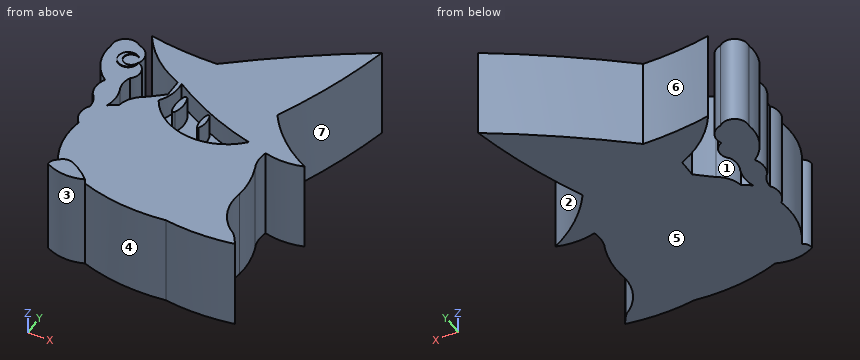
from build123d import *

# Parameters (mm, degrees)
F1_DEPTH = 25.4
F3_DEPTH = 0.254
F5_DEPTH = 6.35
F7_DEPTH = 1.27


with BuildPart() as f1:
    # F0 (on Top) → F1 (new body)
    with BuildSketch(Plane.XY):
        with BuildLine():
            ThreePointArc((25.499046, 10.18772), (37.34433, 7.273723), (49.542308, 7.166576))
            ThreePointArc((49.542308, 7.166576), (59.109263, 6.361494), (68.676218, 7.166576))
            ThreePointArc((68.676218, 7.166576), (67.66707, 8.882251), (66.488296, 10.486125))
            ThreePointArc((66.488296, 10.486125), (61.480718, 16.596846), (60.651142, 24.453597))
            ThreePointArc((60.651142, 24.453597), (60.581585, 29.680598), (59.400324, 34.772847))
            ThreePointArc((59.400324, 34.772847), (58.595793, 37.960262), (58.879148, 41.23541))
            ThreePointArc((58.879148, 41.23541), (64.299362, 40.444263), (69.719575, 41.23541))
            ThreePointArc((69.719575, 41.23541), (61.198485, 47.34438), (54.501284, 55.41135))
            ThreePointArc((54.501284, 55.41135), (61.017596, 71.57709), (65.758646, 88.349566))
            ThreePointArc((65.758646, 88.349566), (48.603509, 77.579957), (32.279015, 65.588541))
            ThreePointArc((32.279015, 65.588541), (22.727137, 66.05081), (13.27099, 67.476757))
            ThreePointArc((13.27099, 67.476757), (19.281494, 60.099473), (27.243776, 54.888662))
            Line((27.243776, 54.888662), (27.243776, 49.727544))
            ThreePointArc((27.243776, 49.727544), (24.946398, 47.862182), (22.58618, 46.076994))
            ThreePointArc((22.58618, 46.076994), (19.956312, 43.712231), (18.683871, 40.412351))
            ThreePointArc((18.683871, 40.412351), (17.413772, 39.740532), (16.166251, 39.027661))
            ThreePointArc((16.166251, 39.027661), (16.709722, 42.300567), (16.166251, 45.573473))
            ThreePointArc((16.166251, 45.573473), (15.61028, 48.154032), (16.166251, 50.734591))
            ThreePointArc((16.166251, 50.734591), (17.468425, 54.06764), (15.285085, 56.902759))
            ThreePointArc((15.285085, 56.902759), (15.245628, 60.550066), (12.389823, 62.819161))
            ThreePointArc((12.389823, 62.819161), (8.109951, 63.436313), (6.221656, 59.546258))
            ThreePointArc((6.221656, 59.546258), (6.981172, 52.747617), (11.148616, 47.322601))
            ThreePointArc((11.148616, 47.322601), (10.300829, 44.357989), (10.931111, 41.339643))
            ThreePointArc((10.931111, 41.339643), (12.26077, 39.219384), (12.659186, 36.748603))
            ThreePointArc((12.659186, 36.748603), (11.67473, 33.258245), (13.162711, 29.95103))
            ThreePointArc((13.162711, 29.95103), (13.136507, 21.545797), (16.183855, 13.712387))
            ThreePointArc((16.183855, 13.712387), (15.066637, 12.687257), (14.799166, 11.194767))
            ThreePointArc((14.799166, 11.194767), (20.034555, 9.474147), (25.499046, 10.18772))
        make_face()
    extrude(amount=F1_DEPTH)

    # F2 (on face) → F3 (join)
    with BuildSketch(Plane.XY.offset(25.4)):
        with BuildLine():
            ThreePointArc((15.285085, 56.902759), (11.304381, 56.052081), (14.373336, 58.726248))
            ThreePointArc((14.373336, 58.726248), (10.050782, 55.425279), (15.285085, 56.902759))
        make_face()
    extrude(amount=F3_DEPTH)

    # F4 (on face) → F5 (cut)
    with BuildSketch(Plane.XY.offset(25.4)):
        with BuildLine():
            ThreePointArc((28.30782, 54.837245), (28.14811, 50.533264), (26.335881, 46.626144))
            ThreePointArc((26.335881, 46.626144), (38.875379, 37.904283), (53.269263, 43.01564))
            ThreePointArc((53.269263, 43.01564), (40.303335, 47.901924), (28.30782, 54.837245))
        make_face()
        with BuildLine():
            ThreePointArc((39.436687, 42.002268), (39.013767, 44.590738), (39.47692, 47.172312))
            ThreePointArc((39.47692, 47.172312), (39.828965, 47.383895), (40.181011, 47.172312))
            ThreePointArc((40.181011, 47.172312), (40.563597, 44.57128), (39.919492, 42.022385))
            ThreePointArc((39.919492, 42.022385), (39.683239, 41.888733), (39.436687, 42.002268))
        make_face(mode=Mode.SUBTRACT)
        with BuildLine():
            ThreePointArc((31.047942, 44.697933), (30.682425, 47.680975), (31.24911, 50.632417))
            ThreePointArc((31.24911, 50.632417), (31.716176, 50.937117), (32.15437, 50.592184))
            ThreePointArc((32.15437, 50.592184), (32.630986, 47.625359), (31.953201, 44.697933))
            ThreePointArc((31.953201, 44.697933), (31.500571, 44.415393), (31.047942, 44.697933))
        make_face(mode=Mode.SUBTRACT)
    extrude(amount=-F5_DEPTH, mode=Mode.SUBTRACT)

    # F6 (on face) → F7 (join)
    with BuildSketch(Plane.XY.offset(25.4)):
        with BuildLine():
            ThreePointArc((19.70306, 14.540644), (17.799455, 14.738373), (16.183855, 13.712387))
            ThreePointArc((16.183855, 13.712387), (15.066637, 12.687257), (14.799166, 11.194767))
            ThreePointArc((14.799166, 11.194767), (20.034555, 9.474147), (25.499046, 10.18772))
            ThreePointArc((25.499046, 10.18772), (22.810777, 12.643433), (19.70306, 14.540644))
        make_face()
    extrude(amount=F7_DEPTH)


solid = f1.part
Input: part model. Units: mm. Frame: model coordinates. Face numbers are marked on the shaded views. A direction names the side the tool comes from. Give positions to 0.01 mm unless a question says otherwise; leave off trailing zeros. Write each loop counter-clockwise with the first axis right and the second up, starting at its lowest first coordinate (ties: lowest second). Pieces come first, ordered by that corner, then holes. Notation, with made-up numbers: M 48.5,36 L 69.5,36 A27 ccw 69.5,54 Z; hole C 66,87.5 d9. An arc over 180 degrees is marked long. Write item = value, one per line. Start each with the question number.
1) Material intervals for line 1 along Z through (x, y) = (30, 65.5); line 2 along X through (y, z) = (53.5, 9.5); line 3 along X through (y, z) = (21.5, 8.75), sorted ascending. Write a range as [from, to].
2) Reachability of the marked faces 1, 2 and 3 from +Z, -Z, +X, -X, +Y, -Y: full face, straight path, thin tool, end or side. Return the list, or none.
3) First-contact query: pin 1 Ø12 at (y, z) = (56, 9.5) entering from +X; pin 2 Ø3 at (x, z) = (25, 15) entering from -Y; pin 3 Ø5 at (x, y) = (41, 48) entering from +Z. Flat tips, straight axial feed; report the tip coordinate or a pass-through.
4) Cut plane B-B on z = 14.75. Return the cut outline in (x, y), then the cut area to 3 significant figures.
5) Cut plane C-C on x = 35. Return the cut outline in (y, z).
6) Draft query along X for the marked faces 4, 5, 6 and 7. Return one class per face: +X half, -X half, draft (parallel to the pull), parting line (faces both ways), or undercut.
7) Cut plane A-A on x = 64. Return the cut outline in (y, z), then the cut area to 3 significant figures.
8) Cut plane D-D on z = 23.25. Count the separate pieces of the cut face and the enclosed holes in it, then the cut area to 3 significant figures.
Solved:
q1.line_1 = [0, 25.4]
q1.line_2 = [6.71, 17.5], [27.24, 55.79]
q1.line_3 = [13.15, 60.42]
q2.face_1 = +Z, -Z
q2.face_2 = +Z, -Z, +X
q2.face_3 = +Z, -Z, -Y
q3.pin_1 = 58.59
q3.pin_2 = 9.63
q3.pin_3 = 25.4
q4.outline = M 6.22,59.55 A12.74 ccw 11.15,47.32 A6.43 ccw 10.93,41.34 A6.29 cw 12.66,36.75 A5.3 ccw 13.16,29.95 A22.6 ccw 16.18,13.71 A2.37 ccw 14.8,11.19 A12.42 ccw 25.5,10.19 A52.6 ccw 49.54,7.17 A57.25 ccw 68.68,7.17 A19.5 ccw 66.49,10.49 A13.78 cw 60.65,24.45 A24.4 ccw 59.4,34.77 A9.9 cw 58.88,41.24 A18.96 ccw 69.72,41.24 A41.08 cw 54.5,55.41 A161.93 ccw 65.76,88.35 A277.7 ccw 32.28,65.59 A94.43 cw 13.27,67.48 A31.05 ccw 27.24,54.89 L 27.24,49.73 A85.97 cw 22.59,46.08 A7.59 ccw 18.68,40.41 A44.06 ccw 16.17,39.03 A10.13 ccw 16.17,45.57 A6.27 cw 16.17,50.73 A3.64 ccw 15.29,56.9 A4.24 ccw 12.39,62.82 A3.66 ccw Z
q4.area = 3,020 mm2
q5.outline = M 7.62,0 L 67.72,0 L 67.72,25.4 L 50.65,25.4 L 50.65,19.05 L 38.91,19.05 L 38.91,25.4 L 7.62,25.4 Z
q6.face_4 = undercut
q6.face_5 = draft
q6.face_6 = undercut
q6.face_7 = +X half
q7.outline = M 6.57,0 L 12.64,0 L 12.64,25.4 L 6.57,25.4 Z; M 40.45,0 L 44.96,0 L 44.96,25.4 L 40.45,25.4 Z; M 81.29,0 L 87.32,0 L 87.32,25.4 L 81.29,25.4 Z
q7.area = 422 mm2
q8.separate_pieces = 3
q8.enclosed_holes = 1
q8.area = 2,820 mm2
